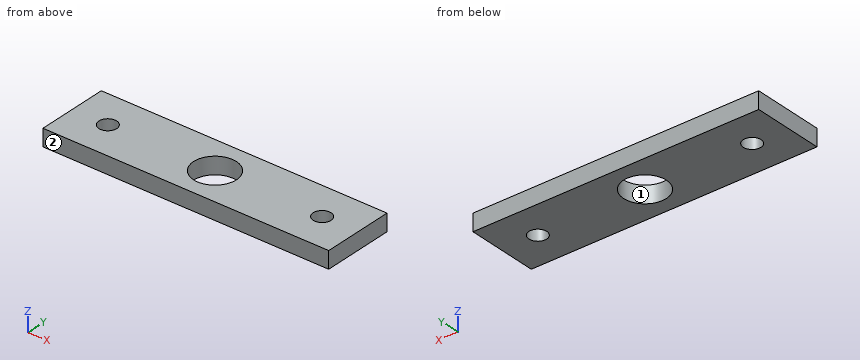
from build123d import *

# Parameters (mm, degrees)
SKETCH1_W           = 80
SKETCH1_H           = 20
SKETCH1_R           = 2.5
SKETCH1_R_2         = 6
BOSS_EXTRUDE1_DEPTH = 4.76


with BuildPart() as part:
    # Sketch1 → Boss-Extrude1 (new body)
    with BuildSketch(Plane.XY.offset(4.76)):
        with Locations((40, 10)):
            Rectangle(SKETCH1_W, SKETCH1_H)
        with Locations(Location((10, 10, 0), (0, 0, 180))):
            Circle(SKETCH1_R, mode=Mode.SUBTRACT)
        with Locations(Location((70, 10, 0), (0, 0, 180))):
            Circle(SKETCH1_R, mode=Mode.SUBTRACT)
        with Locations(Location((40, 10, 0), (0, 0, 180))):
            Circle(SKETCH1_R_2, mode=Mode.SUBTRACT)
    extrude(amount=-BOSS_EXTRUDE1_DEPTH)


solid = part.part
Work out the finished part from the listing and answer in its coordinate system (mm). Face numbers are marked on the shaded views. Round coordinates to 2 decimals unless told otherwise and drop trailing zeros. Write each loop counter-clockwise with the first axis right and the second up, starting at its lowest first coordinate (ties: lowest second). Pieces come first, ordered by that corner, then holes. Notation, with made-up numbers: (-33.5, 11.5) -> (-19.5, 11.5) arc R12 cw to (-19.5, 19.5) -> close; hole circle Ø8 at (43, 74.5). An arc over 180 degrees is marked (long way). Answer as CSV lines item,"result". Start each with the question number.
(1) The part is cut by section C-C, the plane z = 2.25. Give the vertices of the cut face in (x, y).
(2) Find the intervals of material crossed by probe 1 along X at (y, z) = (10, 2.7); probe 2 along Y at (x, z) = (40, 1.85); probe 3 along X at (y, z) = (8.5, 0.45), in increasing order.
(3) The part is cut by section B-B, the plane y = 10. Give the vertices of the cut face in (x, z), then the cut area to 3 significant figures.
(4) The part is cut by section A-A, the plane x = 70. Give the vertices of the cut face in (y, z).
(5) The part is cut by section D-D, the plane y = 13.5. Give the vertices of the cut face in (x, z).
(6) The mould has two halves that part along X. Classify the marked faces 1 and 2: +X half, -X half, draft (parallel to the pull), parting line (faces both ways), or undercut.
(7) Each of these flat-tipped pins is pushed along its axis until it touches: pin 1 (6 mm diameter, centred on x = 38.5, y = 6.5, fed in from -Z); pin 2 (3 mm diameter, centred on x = 10, y = 10, fed in from -Z). Where does it stop, or does it pass through?
Output values:
1,outline,"(0, 0) -> (80, 0) -> (80, 20) -> (0, 20) -> close; hole circle Ø5 at (10, 10); hole circle Ø12 at (40, 10); hole circle Ø5 at (70, 10)"
2,probe 1,"x = 0 to 7.5, 12.5 to 34, 46 to 67.5, 72.5 to 80"
2,probe 2,"y = 0 to 4, 16 to 20"
2,probe 3,"x = 0 to 8, 12 to 34.19, 45.81 to 68, 72 to 80"
3,outline,"(0, 0) -> (7.5, 0) -> (7.5, 4.76) -> (0, 4.76) -> close; (12.5, 0) -> (34, 0) -> (34, 4.76) -> (12.5, 4.76) -> close; (46, 0) -> (67.5, 0) -> (67.5, 4.76) -> (46, 4.76) -> close; (72.5, 0) -> (80, 0) -> (80, 4.76) -> (72.5, 4.76) -> close"
3,area,"276 mm²"
4,outline,"(0, 0) -> (7.5, 0) -> (7.5, 4.76) -> (0, 4.76) -> close; (12.5, 0) -> (20, 0) -> (20, 4.76) -> (12.5, 4.76) -> close"
5,outline,"(0, 0) -> (35.13, 0) -> (35.13, 4.76) -> (0, 4.76) -> close; (44.87, 0) -> (80, 0) -> (80, 4.76) -> (44.87, 4.76) -> close"
6,face 1,"undercut"
6,face 2,"draft"
7,pin 1,"stops at z = 0"
7,pin 2,"passes through"
